Can you work these out from the model? Positions are in its coordinate system, mm. A direction names the side the tool comes from. Coordinates: 2 decimals unless noted, no trailing zeros. Order: outer loops, then holes, each group sorted by start corner. A loop starts at its lowest first (then second) coordinate and runs counter-clockwise, first axis right, second up. Notation, with made-up numbers: M -12.5,2.5 L 39.5,2.5 A24 ccw 39.5,26.5 Z; hole C 48.5,89 d7. An arc over 180 degrees is marked long. Answer as CSV lines item,"result". Start each with the question number.
1. I need wall thicknesses on line 1 along X through (y, z) = (1.5, 69.5); line 2 along Z through (x, y) = (25.5, 1.8); line 3 along X through (y, z) = (1.35, -56.5). Which ranges of each line are inside material? Lowest first, please. Write a range as from..to.
2. If we section it at D-D (z = 17): List the corners of the cut face in (x, y) for me.
3. On a 3-axis mill with a long thin cutter (end or side, diameter ignored), from which of +Z, -Z, +X, -X, +Y, -Y can I reach the whole of each face in a straight line? I mean faces 1 (the face through (3.291, 0.986, -86.938)), 2 (the face through (-33.52, 1.51, 21.83)), 3 (the face through (38.25, 1.49, 54.11)), 4 (the face through (54.11, 1.49, -38.25)). Say none if no direction works.
4. If we section it at A-A (y = 1.6): List the corners of the cut face in (x, z) for me.
5. Will these pins go through, and if not, where does the flat tip stop? pin 1 (6 mm diameter, centred on x = -53, z = -25.5, fed in from -Y); pin 2 (6 mm diameter, centred on x = -13.5, z = -56, fed in from +Y); pin 3 (2 mm diameter, centred on x = -27.5, z = 69.5, fed in from +Y); pin 4 (1 mm diameter, centred on y = 1.5, z = -16.5, fed in from +X).
6. If we section it at B-B (x = -40): List the corners of the cut face in (y, z) for me, plus the area to 3 significant figures.
7. If we section it at C-C (z = -15): List the corners of the cut face in (x, y) for me.
8. If we mould it in two halves opening along X, with no side actions, what happens to faces 5 (the face through (-54.11, 1.51, -38.25)), 6 (the face through (-1, 2, 32)), 7 (the face through (-38.756, 1.507, 54.434))? For each: released by +X, released by -X, zero draft, split by the parting line, or undercut.
```python
from build123d import *

# Parameters (mm, degrees)
RESSALTO_EXTRUS_O1_DEPTH = 2
ESBO_O3_W                = 55
ESBO_O3_H                = 55
CORTE_EXTRUS_O1_DEPTH    = 1
CORTE_EXTRUS_O2_DEPTH    = 1
ESPELHAR1_START          = 1
ESPELHAR1_DEPTH          = 1
ESBO_O5_R                = 1.65
CORTE_EXTRUS_O3_DEPTH    = 2


# Read off the part's stored shape, not the designer's step: Espelhar1
with BuildPart() as part:
    # Esboço2 → Ressalto-extrusão1 (new body)
    with BuildSketch(Plane(origin=(0, 0, 0), x_dir=(1, 0, 0), z_dir=(0, 1, 0))):
        with BuildLine():
            Line((-37, -78.74007874), (37, -78.74007874))
            ThreePointArc((37, -78.74007874), (0, 87), (-37, -78.74007874))
        make_face()
    extrude(amount=RESSALTO_EXTRUS_O1_DEPTH)

    # Esboço3 → Corte-extrusão1 (cut)
    with BuildSketch(Plane(origin=(0, 2, 0), x_dir=(1, 0, 0), z_dir=(0, 1, 0))):
        Rectangle(ESBO_O3_W, ESBO_O3_H)
    extrude(amount=-CORTE_EXTRUS_O1_DEPTH, mode=Mode.SUBTRACT)

    # Esboço4 → Corte-extrusão2 (cut)
    with BuildSketch(Plane(origin=(0, 2, 0), x_dir=(1, 0, 0), z_dir=(0, 1, 0))):
        Polygon((-0.472209327, 47.167542), (-42.60471375, 20.244465077), (-69.527790673, 62.376969501), (-27.39528625, 89.300046424), align=None)
        Polygon((-20.244465077, -42.60471375), (-47.167542, -0.472209327), (-89.300046424, -27.39528625), (-62.376969501, -69.527790673), align=None)
    extrude(amount=-CORTE_EXTRUS_O2_DEPTH, mode=Mode.SUBTRACT)

    # Espelhar1 outline → Espelhar1 (cut)
    with BuildSketch(Plane(origin=(0, 0, 0), x_dir=(1, 0, 0), z_dir=(0, 1, 0)).offset(ESPELHAR1_START)):
        with BuildLine():
            Line((42.60471375, 20.244465077), (65.936611163, 56.757055141))
            ThreePointArc((65.936611163, 56.757055141), (46.846153846, 73.310557697), (23.80410674, 83.680132064))
            Line((23.80410674, 83.680132064), (0.472209327, 47.167542))
            Line((0.472209327, 47.167542), (42.60471375, 20.244465077))
        make_face()
        with BuildLine():
            ThreePointArc((56.757055141, -65.936611163), (73.310557697, -46.846153846), (83.680132064, -23.80410674))
            Line((83.680132064, -23.80410674), (47.167542, -0.472209327))
            Line((47.167542, -0.472209327), (20.244465077, -42.60471375))
            Line((20.244465077, -42.60471375), (56.757055141, -65.936611163))
        make_face()
    extrude(amount=ESPELHAR1_DEPTH, mode=Mode.SUBTRACT)

    # Esboço5 → Corte-extrusão3 (cut)
    with BuildSketch(Plane(origin=(0, 2, 0), x_dir=(1, 0, 0), z_dir=(0, 1, 0))):
        with Locations(Location((-27.5, -69.5, 0), (0, 0, 270))):
            Circle(ESBO_O5_R)
        with Locations(Location((27.5, -69.5, 0), (0, 0, 270))):
            Circle(ESBO_O5_R)
    extrude(amount=-CORTE_EXTRUS_O3_DEPTH, mode=Mode.SUBTRACT)


solid = part.part
```
Solved:
1,line 1,"-52.33..-29.15, -25.85..25.85, 29.15..52.33"
1,line 2,"-31.17..-27.5, 27.5..34.38, 45.96..78.74"
1,line 3,"-66.16..-65.77, -6.44..6.44, 65.77..66.16"
2,outline,"M -85.32,0 L 85.32,0 L 85.32,2 L 73.03,2 L 73.03,1 L 36.61,1 L 36.61,2 L 27.5,2 L 27.5,1 L -27.5,1 L -27.5,2 L -36.61,2 L -36.61,1 L -73.03,1 L -73.03,2 L -85.32,2 Z"
3,face 1,"+Y, -Y"
3,face 2,"+Y"
3,face 3,"+X, +Y"
3,face 4,"-Z, +Y"
4,outline,"M -83.68,23.8 A87 ccw -65.94,-56.76 L -42.6,-20.24 L -0.47,-47.17 L -23.8,-83.68 A87 ccw 23.8,-83.68 L 0.47,-47.17 L 42.6,-20.24 L 65.94,-56.76 A87 ccw 83.68,23.8 L 47.17,0.47 L 20.24,42.6 L 56.76,65.94 A87 ccw 37,78.74 L -37,78.74 A87 ccw -56.76,65.94 L -20.24,42.6 L -47.17,0.47 Z; hole C -27.5,69.5 d3.3; hole M -27.5,-27.5 L 27.5,-27.5 L 27.5,27.5 L -27.5,27.5 Z; hole C 27.5,69.5 d3.3"
5,pin 1,"y = 0"
5,pin 2,"y = 1"
5,pin 3,"through"
5,pin 4,"x = 85.52"
6,outline,"M 0,-77.26 L 1,-77.26 L 1,-21.91 L 2,-21.91 L 2,11.69 L 1,11.69 L 1,55.23 L 2,55.23 L 2,77.26 L 0,77.26 Z"
6,area,"210 mm²"
7,outline,"M -85.7,0 L 85.7,0 L 85.7,2 L 27.5,2 L 27.5,1 L -27.5,1 L -27.5,2 L -85.7,2 Z"
8,face 5,"undercut"
8,face 6,"zero draft"
8,face 7,"released by -X"
